```python
from build123d import *

# Parameters (mm, degrees)
F0_R     = 2.825681
F0_R_2   = 4.106175
F0_R_3   = 2.633884
F0_R_4   = 1.979989
F0_R_5   = 2.894334
F0_R_6   = 3.256127
F0_R_7   = 2.425647
F0_R_8   = 2.316591
F0_R_9   = 3.635961
F0_R_10  = 2.934407
F0_R_11  = 3.112248
F0_R_12  = 2.316604
F0_R_13  = 2.558261
F1_DEPTH = 2.794


with BuildPart() as f1:
    # F0 (on Top) → F1 (new body)
    with BuildSketch(Plane.XY):
        with BuildLine():
            Line((77.282588, -22.826083), (77.282588, 22.826083))
            Line((77.282588, 22.826083), (61.630418, 22.826083))
            Line((61.630418, 22.826083), (-62.282588, 22.826083))
            Line((-62.282588, 22.826083), (-62.282588, 92.826083))
            ThreePointArc((-62.282588, 92.826083), (-69.782588, 119.46184), (-77.282588, 92.826083))
            Line((-77.282588, 92.826083), (-77.282588, 22.826083))
            Line((-77.282588, 22.826083), (-77.282588, -22.826083))
            Line((-77.282588, -22.826083), (-77.282588, -92.826083))
            ThreePointArc((-77.282588, -92.826083), (-69.782588, -118.714864), (-62.282588, -92.826083))
            Line((-62.282588, -92.826083), (-62.282588, -22.826083))
            Line((-62.282588, -22.826083), (61.630418, -22.826083))
            Line((61.630418, -22.826083), (77.282588, -22.826083))
        make_face()
        with Locations((-75.795345, -111.477017)):
            Circle(F0_R, mode=Mode.SUBTRACT)
        with Locations((-66.388763, -112.200603)):
            Circle(F0_R_2, mode=Mode.SUBTRACT)
        with Locations((-77.242516, -99.899687)):
            Circle(F0_R_3, mode=Mode.SUBTRACT)
        with Locations((-69.782588, -99.176109)):
            Circle(F0_R_4, mode=Mode.SUBTRACT)
        with Locations((-77.242516, 100.171089)):
            Circle(F0_R_5, mode=Mode.SUBTRACT)
        with Locations((-66.388763, 100.171089)):
            Circle(F0_R_6, mode=Mode.SUBTRACT)
        with Locations((-77.242516, 108.492292)):
            Circle(F0_R_5, mode=Mode.SUBTRACT)
        with Locations((-69.782588, 109.939463)):
            Circle(F0_R_7, mode=Mode.SUBTRACT)
        with BuildLine():
            Line((61.630418, 22.826083), (77.282588, 22.826083))
            Line((77.282588, 22.826083), (77.282588, 92.826083))
            ThreePointArc((77.282588, 92.826083), (69.456503, 119.065138), (61.630418, 92.826083))
            Line((61.630418, 92.826083), (61.630418, 22.826083))
        make_face()
        with Locations((62.409062, 100.532882)):
            Circle(F0_R_8, mode=Mode.SUBTRACT)
        with Locations((60.961891, 108.854085)):
            Circle(F0_R_9, mode=Mode.SUBTRACT)
        with Locations((74.348181, 100.171089)):
            Circle(F0_R_10, mode=Mode.SUBTRACT)
        with Locations((74.348181, 109.939463)):
            Circle(F0_R_10, mode=Mode.SUBTRACT)
        with BuildLine():
            Line((77.282588, -92.826083), (77.282588, -22.826083))
            Line((77.282588, -22.826083), (61.630418, -22.826083))
            Line((61.630418, -22.826083), (61.630418, -92.826083))
            ThreePointArc((61.630418, -92.826083), (69.456503, -118.891843), (77.282588, -92.826083))
        make_face()
        with Locations((64.218014, -112.200603)):
            Circle(F0_R_11, mode=Mode.SUBTRACT)
        with Locations((74.348181, -111.477017)):
            Circle(F0_R_12, mode=Mode.SUBTRACT)
        with Locations((62.770844, -97.728938)):
            Circle(F0_R_13, mode=Mode.SUBTRACT)
        with Locations((74.348181, -96.64356)):
            Circle(F0_R_10, mode=Mode.SUBTRACT)
    extrude(amount=F1_DEPTH)


solid = f1.part
```
Read the model definition and answer for the solid it produces. Units are mm, in the model's axes. Give positions to 0.01 mm unless a question says otherwise; leave off trailing zeros. Loops run counter-clockwise (first coordinate to the right, second up) from the corner with the lowest first, then second, coordinate; pieces in that order, holes last.
Item 1: The part is cut by section C-C (x = -9.5). Write down the section's boundary in (y, z), and give its area (3 significant figures).
Item 2: The part is cut by section B-B (z = 1.8). Give the number of separate pieces and of enclosed holes in the cut face, and give its area (3 significant figures).
Item 3: Find the intervals of material crossed by line 1 along X through (y, z) = (-40.5, 1.9); line 2 along Y through (x, z) = (57, 1.45); line 3 along Y through (x, z) = (-38, 2.45), in increasing order.
Item 4: Each of these flat-tipped pins is pushed along its axis until it touches: pin 1 Ø1.4 at (y, z) = (32.5, 1) entering from +X; pin 2 Ø1.4 at (x, z) = (-21, 1) entering from +Y; pin 3 Ø1.4 at (y, z) = (29.5, 1) entering from -X. Where does it stop, or does it pass through?
Item 5: The mould has two halves that part along Y. Classify faces 1 (the flat face through (6, 1, 2.794)), 2 (the cylindrical face through (-77.62, 103.04, 1.38)): released by +Y, released by -Y, zero draft, split by the parting line, or undercut.
Item 6: The part is cut by section D-D (y = -8). Write down the section's boundary in (x, z), and give its area (3 significant figures).
Item 7: The part is cut by section A-A (y = 79). Write down the section's boundary in (x, z).
Taken from the geometry:
1. outline: (-22.83, 0) - (22.83, 0) - (22.83, 2.79) - (-22.83, 2.79) - close
1. area: 128 mm2
2. separate pieces: 1
2. enclosed holes: 16
2. area: 13,400 mm2
3. line 1: x = -77.28 to -62.28, 61.63 to 77.28
3. line 2: y = -111.52 to -97.85, -22.83 to 22.83, 97.78 to 111.77
3. line 3: y = -22.83 to 22.83
4. pin 1: stops at x = 77.28
4. pin 2: stops at y = 22.83
4. pin 3: stops at x = -77.28
5. face 1: zero draft
5. face 2: undercut
6. outline: (-77.28, 0) - (77.28, 0) - (77.28, 2.79) - (-77.28, 2.79) - close
6. area: 432 mm2
7. outline: (-77.28, 0) - (-62.28, 0) - (-62.28, 2.79) - (-77.28, 2.79) - close; (61.63, 0) - (77.28, 0) - (77.28, 2.79) - (61.63, 2.79) - close
